Could you check a few things on this model? Use its own coordinates, in mm. Coordinates: 2 decimals unless noted, no trailing zeros. Loops run counter-clockwise (first coordinate to the right, second up) from the corner with the lowest first, then second, coordinate; pieces in that order, holes last. Notation, with made-up numbers: (2, -24.75) - (24, -24.75) arc R32 ccw to (24, 7.25) - close; hole circle Ø9 at (39.25, 25.25). An arc over 180 degrees is marked (long way). Use CSV: the item, a comma, the result in double quotes.
from build123d import *

# Parameters (mm, degrees)
SKETCH1_W           = 300
SKETCH1_H           = 15
BOSS_EXTRUDE1_DEPTH = 15
SKETCH2_W           = 300
SKETCH2_H           = 12.5
CUT_EXTRUDE2_DEPTH  = 12.5
SKETCH3_R           = 5
BOSS_EXTRUDE2_DEPTH = 100


with BuildPart() as part:
    # Sketch1 → Boss-Extrude1 (new body)
    with BuildSketch(Plane(origin=(0, 0, 0), x_dir=(1, 0, 0), z_dir=(0, 1, 0))):
        Rectangle(SKETCH1_W, SKETCH1_H)
    extrude(amount=BOSS_EXTRUDE1_DEPTH)

    # Sketch2 → Cut-Extrude2 (cut)
    with BuildSketch(Plane(origin=(0, 0, 0), x_dir=(1, 0, 0), z_dir=(0, 1, 0))):
        Rectangle(SKETCH2_W, SKETCH2_H)
    extrude(amount=CUT_EXTRUDE2_DEPTH, mode=Mode.SUBTRACT)

    # Sketch3 → Boss-Extrude2 (add)
    with BuildSketch(Plane(origin=(0, 15, 0), x_dir=(1, 0, 0), z_dir=(0, 1, 0))):
        Circle(SKETCH3_R)
    extrude(amount=BOSS_EXTRUDE2_DEPTH)


solid = part.part
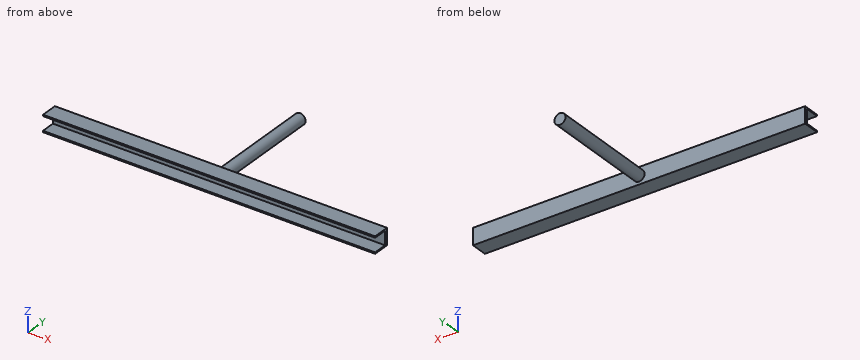
(1) Suppose I cut it at D-D (x = -39). Write out the boundary of the cut face in (y, z).
Computed:
outline,"(0, -7.5) - (15, -7.5) - (15, 7.5) - (0, 7.5) - (0, 6.25) - (12.5, 6.25) - (12.5, -6.25) - (0, -6.25) - close"
(2) Suppose I cut it at B-B (z = 0). Write out the boundary of the cut face in (x, y).
Computed:
outline,"(-150, 12.5) - (150, 12.5) - (150, 15) - (5, 15) - (5, 115) - (-5, 115) - (-5, 15) - (-150, 15) - close"
(3) Suppose I cut it at C-C (y = 58). Write out the boundary of the cut face in (x, z), plus the area to 3 significant figures.
Computed:
outline,"circle Ø10 at (0, 0)"
area,"78.5 mm²"
(4) Suppose I cut it at A-A (x = 0). Write out the boundary of the cut face in (y, z), plus the area to 3 significant figures.
Computed:
outline,"(0, -7.5) - (15, -7.5) - (15, -5) - (115, -5) - (115, 5) - (15, 5) - (15, 7.5) - (0, 7.5) - (0, 6.25) - (12.5, 6.25) - (12.5, -6.25) - (0, -6.25) - close"
area,"1,070 mm²"
(5) Please list where these lines run through material, in increasing order: line 1 (Y direction, x = -114, z = -5.5); line 2 (X direction, y = 65.5, z = -0.5).
Computed:
line 1,"y = 12.5 to 15"
line 2,"x = -4.97 to 4.97"
(6) Will these pins go through, and if not, where does the flat tip stop? pin 1 (6 mm diameter, centred on x = -4, y = 93.5, fed in from -Z); pin 2 (1.5 mm diameter, centred on y = 89.5, z = -0.5, fed in from +X); pin 3 (5 mm diameter, centred on x = -14, z = -4.5, fed in from -Y); pin 4 (1.5 mm diameter, centred on y = 67, z = -3.5, fed in from +X).
Computed:
pin 1,"stops at z = -4.9"
pin 2,"stops at x = 5"
pin 3,"stops at y = 0"
pin 4,"stops at x = 4.18"
